```python
from build123d import *

# Parameters (mm, degrees)
SKETCH1_R                = 2.05
BOSS_EXTRUDE1_DEPTH      = 6
CUT_EXTRUDE1_DEPTH       = 4
BOSS_EXTRUDE2_DEPTH      = 12
BOSS_EXTRUDE2_DEPTH_BACK = 1
SKETCH4_R                = 8.5
SKETCH4_R_2              = 2.05
CHAMFER3_SIZE            = 0.8


with BuildPart() as part:
    # Sketch1 → Boss-Extrude1 (new body)
    with BuildSketch(Plane.XY):
        with BuildLine():
            Line((-52.397368877, 8.273451517), (-43.689164944, 12.627553483))
            ThreePointArc((-43.689164944, 12.627553483), (-40.86217617, 13.652236863), (-37.875388203, 14))
            Line((-37.875388203, 14), (37.875388203, 14))
            ThreePointArc((37.875388203, 14), (40.86217617, 13.652236863), (43.689164944, 12.627553483))
            Line((43.689164944, 12.627553483), (52.397368877, 8.273451517))
            ThreePointArc((52.397368877, 8.273451517), (54.728318318, 7.650368424), (57.116243367, 7.995870664))
            ThreePointArc((57.116243367, 7.995870664), (67.602631123, -3.801315562), (51.873049489, -2.490517092))
            ThreePointArc((51.873049489, -2.490517092), (50.716696252, -0.372875708), (48.819660113, 1.118033989))
            Line((48.819660113, 1.118033989), (40.11145618, 5.472135955))
            ThreePointArc((40.11145618, 5.472135955), (39.024152805, 5.866244947), (37.875388203, 6))
            Line((37.875388203, 6), (-37.875388203, 6))
            ThreePointArc((-37.875388203, 6), (-39.024152805, 5.866244947), (-40.11145618, 5.472135955))
            Line((-40.11145618, 5.472135955), (-48.819660113, 1.118033989))
            ThreePointArc((-48.819660113, 1.118033989), (-50.716696252, -0.372875708), (-51.873049489, -2.490517092))
            ThreePointArc((-51.873049489, -2.490517092), (-67.602631123, -3.801315562), (-57.116243367, 7.995870664))
            ThreePointArc((-57.116243367, 7.995870664), (-54.728318318, 7.650368424), (-52.397368877, 8.273451517))
        make_face()
        with Locations((-60, 0)):
            Circle(SKETCH1_R, mode=Mode.SUBTRACT)
        with Locations((60, 0)):
            Circle(SKETCH1_R, mode=Mode.SUBTRACT)
    extrude(amount=BOSS_EXTRUDE1_DEPTH)

    # Sketch3 → Cut-Extrude1 (cut)
    with BuildSketch(Plane.XY.offset(6)):
        Polygon((-60, 4.099186911), (-63.55, 2.049593456), (-63.55, -2.049593456), (-60, -4.099186911), (-56.45, -2.049593456), (-56.45, 2.049593456), align=None)
        Polygon((60, 4.099186911), (56.45, 2.049593456), (56.45, -2.049593456), (60, -4.099186911), (63.55, -2.049593456), (63.55, 2.049593456), align=None)
    extrude(amount=-CUT_EXTRUDE1_DEPTH, mode=Mode.SUBTRACT)

    # Sketch4 → Boss-Extrude2 (add, two sides: drawn at the far end of the back side and taken through both)
    with BuildSketch(Plane(origin=(0, 0, 0), x_dir=(-1, 0, 0), z_dir=(0, 0, -1)).offset(-BOSS_EXTRUDE2_DEPTH_BACK)):
        with Locations((-60, 0)):
            Circle(SKETCH4_R)
        with Locations((-60, 0)):
            Circle(SKETCH4_R_2, mode=Mode.SUBTRACT)
    extrude(amount=BOSS_EXTRUDE2_DEPTH + BOSS_EXTRUDE2_DEPTH_BACK)

    # Chamfer3
    # the kernel refuses this chamfer: 0.8 mm, written as the material it adds along each edge
    # the kernel refuses this chamfer: 0.8 mm, written as the material it takes off along each edge
    with BuildSketch(Plane(origin=(37.875388203, 1, 0), x_dir=(0.44721359549995965, 0.894427190999915, 0), z_dir=(0.894427190999915, -0.44721359549995965, 0))) as chamfer3_2_piece_1:
        Polygon((5, CHAMFER3_SIZE), (5 + CHAMFER3_SIZE, 0), (5, 0), align=None)
    revolve(axis=Axis((37.875388203, 1, 0), (0, 0, 1)), revolution_arc=26.565051177, mode=Mode.SUBTRACT)
    with BuildSketch(Plane(origin=(48.819660113, 1.118033989, 0), x_dir=(-0.012296529840444168, -0.024593059680888388, 0.9996219169112966), z_dir=(-0.8944271909999163, 0.44721359549995715, 0)), Plane(origin=(-40.11145618, 5.472135955, 0), x_dir=(0.01229652984044405, -0.02459305968088818, 0.9996219169112966), z_dir=(-0.8944271909999165, -0.4472135954999568, 0)), Plane(origin=(43.689164944, 12.627553483, 0), x_dir=(0.012296529840444093, 0.02459305968088816, 0.9996219169112966), z_dir=(0.8944271909999156, -0.44721359549995837, 0)), Plane(origin=(48.819660113, 1.118033989, 6), x_dir=(0.4470445116024604, 0.8940890232049228, 0.02749587661058619), z_dir=(-0.8944271909999163, 0.44721359549995715, 0)), Plane(origin=(-40.11145618, 5.472135955, 6), x_dir=(-0.4470445116024601, 0.8940890232049231, 0.02749587661058619), z_dir=(-0.8944271909999165, -0.4472135954999568, 0)), Plane(origin=(43.689164944, 12.627553483, 6), x_dir=(-0.4470445116024617, -0.8940890232049222, 0.027495876610586216), z_dir=(0.8944271909999156, -0.44721359549995837, 0)), Plane(origin=(-52.397368877, 8.273451517, 6), x_dir=(0.44704451160246106, -0.8940890232049225, 0.027495876610586212), z_dir=(0.894427190999916, 0.4472135954999578, 0))) as chamfer3_2_piece_2:
        Polygon((CHAMFER3_SIZE * 0.999621916911, CHAMFER3_SIZE * 0.0274958766106), (-CHAMFER3_SIZE * 0.0274958766106, CHAMFER3_SIZE * 0.999621916911), (0, 0), align=None)
    extrude(amount=9.736067977, mode=Mode.SUBTRACT)
    with BuildSketch(Plane(origin=(37.875388203, 6, 0), x_dir=(0, -0.027495876610586275, 0.9996219169112968), z_dir=(-1, 0, 0)), Plane(origin=(-37.875388203, 14, 0), x_dir=(0, 0.02749587661058735, 0.9996219169112966), z_dir=(1, 0, 0)), Plane(origin=(37.875388203, 6, 6), x_dir=(0, 0.9996219169112968, 0.027495876610586285), z_dir=(-1, 0, 0)), Plane(origin=(-37.875388203, 14, 6), x_dir=(0, -0.9996219169112968, 0.027495876610586226), z_dir=(1, 0, 0))) as chamfer3_2_piece_3:
        Polygon((CHAMFER3_SIZE * 0.999621916911, CHAMFER3_SIZE * 0.0274958766106), (-CHAMFER3_SIZE * 0.0274958766106, CHAMFER3_SIZE * 0.999621916911), (0, 0), align=None)
    extrude(amount=75.750776405, mode=Mode.SUBTRACT)
    with BuildSketch(Plane(origin=(46.13637854, -4.248529157, 0), x_dir=(0.9989622079668251, -0.04554675678954209, 0), z_dir=(-0.04554675678954209, -0.9989622079668251, 0))) as chamfer3_2_piece_4_section:
        Polygon((6, CHAMFER3_SIZE), (6 + CHAMFER3_SIZE, 0), (6, 0), align=None)
    chamfer3_2_piece_4 = revolve(axis=Axis((46.13637854, -4.248529157, 0), (0, 0, 1)), revolution_arc=66.045488886, mode=Mode.PRIVATE)
    chamfer3_2_piece_4 = chamfer3_2_piece_4 - Plane(origin=(60, 0, 0.316419024), x_dir=(-1, 0, 0), z_dir=(0, 0, 1)) * Cylinder(8.5, 28, mode=Mode.PRIVATE)
    add(chamfer3_2_piece_4, mode=Mode.SUBTRACT)
    with BuildSketch(Plane(origin=(-37.875388203, 1, 0), x_dir=(0, 1, 0), z_dir=(1, 0, 0))) as chamfer3_2_piece_5:
        Polygon((5, CHAMFER3_SIZE), (5 + CHAMFER3_SIZE, 0), (5, 0), align=None)
    revolve(axis=Axis((-37.875388203, 1, 0), (0, 0, 1)), revolution_arc=26.565051177, mode=Mode.SUBTRACT)
    with BuildSketch(Plane(origin=(55.08065045, 13.640014663, 0), x_dir=(-0.44721359549995726, -0.8944271909999163, 0), z_dir=(-0.8944271909999163, 0.44721359549995726, 0))) as chamfer3_2_piece_6_section:
        Polygon((6, CHAMFER3_SIZE), (6 + CHAMFER3_SIZE, 0), (6, 0), align=None)
    chamfer3_2_piece_6 = revolve(axis=Axis((55.08065045, 13.640014663, 0), (0, 0, 1)), revolution_arc=66.045488886, mode=Mode.PRIVATE)
    chamfer3_2_piece_6 = chamfer3_2_piece_6 - Plane(origin=(60, 0, 0.316418933), x_dir=(-1, 0, 0), z_dir=(0, 0, 1)) * Cylinder(8.5, 28, mode=Mode.PRIVATE)
    add(chamfer3_2_piece_6, mode=Mode.SUBTRACT)
    with BuildSketch(Plane(origin=(-46.13637854, -4.248529157, 0), x_dir=(-0.4472135954999641, 0.8944271909999129, 0), z_dir=(0.8944271909999129, 0.4472135954999641, 0))) as chamfer3_2_piece_7:
        Polygon((6, CHAMFER3_SIZE), (6 + CHAMFER3_SIZE, 0), (6, 0), align=None)
    revolve(axis=Axis((-46.13637854, -4.248529157, 0), (0, 0, 1)), revolution_arc=46.397181027, mode=Mode.SUBTRACT)
    with BuildSketch(Plane(origin=(-60, 0, 0), x_dir=(0.9561118248619797, -0.29300201084479827, 0), z_dir=(0.29300201084479827, 0.9561118248619797, 0))) as chamfer3_2_piece_8:
        Polygon((8.5 - CHAMFER3_SIZE, 0), (8.5, -CHAMFER3_SIZE), (8.5, 0), align=None)
    revolve(axis=Axis((-60, 0, 0), (0, 0, -1)), revolution_arc=272.794362055, mode=Mode.SUBTRACT)
    with BuildSketch(Plane(origin=(37.875388203, 1, 0), x_dir=(0, 1, 0), z_dir=(-1, 0, 0))) as chamfer3_2_piece_9:
        Polygon((13, -CHAMFER3_SIZE), (13 - CHAMFER3_SIZE, 0), (13, 0), align=None)
    revolve(axis=Axis((37.875388203, 1, 0), (0, 0, -1)), revolution_arc=26.565051177, mode=Mode.SUBTRACT)
    with BuildSketch(Plane(origin=(-55.08065045, 13.640014663, 0), x_dir=(-0.3392654862413453, -0.940690666396464, 0), z_dir=(-0.940690666396464, 0.3392654862413453, 0))) as chamfer3_2_piece_10:
        Polygon((6, CHAMFER3_SIZE), (6 + CHAMFER3_SIZE, 0), (6, 0), align=None)
    revolve(axis=Axis((-55.08065045, 13.640014663, 0), (0, 0, 1)), revolution_arc=46.397181027, mode=Mode.SUBTRACT)
    with BuildSketch(Plane(origin=(-52.397368877, 8.273451517, 0), x_dir=(0.44704451160246106, -0.8940890232049225, -0.027495876610586303), z_dir=(0.894427190999916, 0.4472135954999578, 0))) as chamfer3_2_piece_11:
        Polygon((CHAMFER3_SIZE * 0.999621916911, -CHAMFER3_SIZE * 0.0274958766106), (-CHAMFER3_SIZE * 0.0274958766106, -CHAMFER3_SIZE * 0.999621916911), (0, 0), align=None)
    extrude(amount=9.736067977, mode=Mode.SUBTRACT)
    with BuildSketch(Plane(origin=(-37.875388203, 1, 0), x_dir=(-0.4472135954999576, 0.894427190999916, 0), z_dir=(-0.894427190999916, -0.4472135954999576, 0))) as chamfer3_2_piece_12:
        Polygon((13, -CHAMFER3_SIZE), (13 - CHAMFER3_SIZE, 0), (13, 0), align=None)
    revolve(axis=Axis((-37.875388203, 1, 0), (0, 0, -1)), revolution_arc=26.565051177, mode=Mode.SUBTRACT)
    with BuildSketch(Plane(origin=(37.875388203, 1, 6), x_dir=(0.44721359549995965, 0.894427190999915, 0), z_dir=(0.894427190999915, -0.44721359549995965, 0))) as chamfer3_2_piece_13:
        Polygon((5 + CHAMFER3_SIZE, 0), (5, -CHAMFER3_SIZE), (5, 0), align=None)
    revolve(axis=Axis((37.875388203, 1, 6), (0, 0, 1)), revolution_arc=26.565051177, mode=Mode.SUBTRACT)
    with BuildSketch(Plane(origin=(46.13637854, -4.248529157, 6), x_dir=(0.956111824861979, 0.2930020108448003, 0), z_dir=(0.2930020108448003, -0.956111824861979, 0))) as chamfer3_2_piece_14:
        Polygon((6 + CHAMFER3_SIZE, 0), (6, -CHAMFER3_SIZE), (6, 0), align=None)
    revolve(axis=Axis((46.13637854, -4.248529157, 6), (0, 0, 1)), revolution_arc=46.397181027, mode=Mode.SUBTRACT)
    with BuildSketch(Plane(origin=(-37.875388203, 1, 6), x_dir=(0, 1, 0), z_dir=(1, 0, 0))) as chamfer3_2_piece_15:
        Polygon((5 + CHAMFER3_SIZE, 0), (5, -CHAMFER3_SIZE), (5, 0), align=None)
    revolve(axis=Axis((-37.875388203, 1, 6), (0, 0, 1)), revolution_arc=26.565051177, mode=Mode.SUBTRACT)
    with BuildSketch(Plane(origin=(60, 0, 6), x_dir=(-0.3392654862413484, 0.9406906663964629, 0), z_dir=(-0.9406906663964629, -0.3392654862413484, 0))) as chamfer3_2_piece_16:
        Polygon((8.5 - CHAMFER3_SIZE, 0), (8.5, CHAMFER3_SIZE), (8.5, 0), align=None)
    revolve(axis=Axis((60, 0, 6), (0, 0, -1)), revolution_arc=272.794362055, mode=Mode.SUBTRACT)
    with BuildSketch(Plane(origin=(55.08065045, 13.640014663, 6), x_dir=(-0.44721359549995726, -0.8944271909999163, 0), z_dir=(-0.8944271909999163, 0.44721359549995726, 0))) as chamfer3_2_piece_17:
        Polygon((6 + CHAMFER3_SIZE, 0), (6, -CHAMFER3_SIZE), (6, 0), align=None)
    revolve(axis=Axis((55.08065045, 13.640014663, 6), (0, 0, 1)), revolution_arc=46.397181027, mode=Mode.SUBTRACT)
    with BuildSketch(Plane(origin=(-46.13637854, -4.248529157, 6), x_dir=(-0.4472135954999641, 0.8944271909999129, 0), z_dir=(0.8944271909999129, 0.4472135954999641, 0))) as chamfer3_2_piece_18:
        Polygon((6 + CHAMFER3_SIZE, 0), (6, -CHAMFER3_SIZE), (6, 0), align=None)
    revolve(axis=Axis((-46.13637854, -4.248529157, 6), (0, 0, 1)), revolution_arc=46.397181027, mode=Mode.SUBTRACT)
    with BuildSketch(Plane(origin=(-60, 0, 6), x_dir=(0.9561118248619797, -0.29300201084479827, 0), z_dir=(0.29300201084479827, 0.9561118248619797, 0))) as chamfer3_2_piece_19:
        Polygon((8.5 - CHAMFER3_SIZE, 0), (8.5, CHAMFER3_SIZE), (8.5, 0), align=None)
    revolve(axis=Axis((-60, 0, 6), (0, 0, -1)), revolution_arc=272.794362055, mode=Mode.SUBTRACT)
    with BuildSketch(Plane(origin=(37.875388203, 1, 6), x_dir=(0, 1, 0), z_dir=(-1, 0, 0))) as chamfer3_2_piece_20:
        Polygon((13 - CHAMFER3_SIZE, 0), (13, CHAMFER3_SIZE), (13, 0), align=None)
    revolve(axis=Axis((37.875388203, 1, 6), (0, 0, -1)), revolution_arc=26.565051177, mode=Mode.SUBTRACT)
    with BuildSketch(Plane(origin=(-55.08065045, 13.640014663, 6), x_dir=(-0.3392654862413453, -0.940690666396464, 0), z_dir=(-0.940690666396464, 0.3392654862413453, 0))) as chamfer3_2_piece_21:
        Polygon((6, -CHAMFER3_SIZE), (6 + CHAMFER3_SIZE, 0), (6, 0), align=None)
    revolve(axis=Axis((-55.08065045, 13.640014663, 6), (0, 0, 1)), revolution_arc=46.397181027, mode=Mode.SUBTRACT)
    with BuildSketch(Plane(origin=(-37.875388203, 1, 6), x_dir=(-0.4472135954999576, 0.894427190999916, 0), z_dir=(-0.894427190999916, -0.4472135954999576, 0))) as chamfer3_2_piece_22:
        Polygon((13 - CHAMFER3_SIZE, 0), (13, CHAMFER3_SIZE), (13, 0), align=None)
    revolve(axis=Axis((-37.875388203, 1, 6), (0, 0, -1)), revolution_arc=26.565051177, mode=Mode.SUBTRACT)
    with BuildSketch(Plane(origin=(60, 0, -12), x_dir=(-1, 0, 0), z_dir=(0, -1, 0))) as chamfer3_2_piece_23:
        Polygon((8.5 - CHAMFER3_SIZE, 0), (8.5, -CHAMFER3_SIZE), (8.5, 0), align=None)
    revolve(axis=Axis((60, 0, -12), (0, 0, -1)), mode=Mode.SUBTRACT)


solid = part.part
```
Geometry check sheet. Reference: the model listing, model coordinates, mm. A direction names the side the tool comes from. Give positions to 0.01 mm unless a question says otherwise; leave off trailing zeros. Loops run counter-clockwise (first coordinate to the right, second up) from the corner with the lowest first, then second, coordinate; pieces in that order, holes last. Notation, with made-up numbers: M -22,36.25 L -8,36.25 A20 cw -8,49.25 Z; hole C -1,84 d10. An arc over 180 degrees is marked long. Write item = value, one per line.
(1) Gauge pin test, flat ends, axial feed: pin 1 Ø5.5 at (x, y) = (-60, -0.5) entering from +Z; pin 2 Ø5 at (x, y) = (-52.5, 0) entering from -Z; pin 3 Ø2 at (x, y) = (59, 0) entering from +Z; pin 4 Ø5 at (x, z) = (4.5, 4) entering from -Y. Record the tip position at first contact, or that the pin passes through.
Answer below:
pin_1 = 2
pin_2 = 0
pin_3 = through
pin_4 = 6
(2) Release check for a two-part mould opening along Y. For faces 5 (the face through (-44.581, 3.678, 0.406)), 6 (the face through (58, -2, -12)), 7 (the face through (-63.55, 0, 4)) record: released by +Y, released by -Y, zero draft, split by the parting line, or undercut.
Answer below:
face_5 = released by -Y
face_6 = zero draft
face_7 = undercut
(3) Tool access check on faces 1 (the face through (58.2, -3.06, 4.03)), 2 (the face through (-39.01, 5.87, 2.97)), 3 (the face through (-44.59, 3.69, 5.61)), 4 (the face through (50.6, 0.2, 0.5)). Record the directions out of +Z, -Z, +X, -X, +Y, -Y that give a thin tool (end or side, any length) a straight path to the whole face; none if there is none.
Answer below:
face_1 = +Z
face_2 = +Z, -Z, -Y
face_3 = +Z, -Y
face_4 = -Z, -Y
(4) Sectioned sample at A-A, the plane x = -13. Record the cut outline in (y, z).
Answer below:
outline = M 6,0.8 L 6.8,0 L 13.2,0 L 14,0.8 L 14,5.2 L 13.2,6 L 6.8,6 L 6,5.2 Z
(5) Material ranges on line 1 (X direction, y = 0, z = -3.25); line 2 (Y direction, x = 60, z = -8.5); line 3 (X direction, y = -3, z = 4), recorded low to high. Write a range as [from, to].
Answer below:
line_1 = [51.5, 57.95], [62.05, 68.5]
line_2 = [-8.5, -2.05], [2.05, 8.5]
line_3 = [-67.95, -61.9], [-58.1, -52.05], [52.05, 58.1], [61.9, 67.95]
(6) Sectioned sample at B-B, the plane z = -7.75. Record the cut outline in (x, y).
Answer below:
outline = C 60,0 d17; hole C 60,0 d4.1
